Autodesk Inventor part; units mm, degrees
ref_plane "Work Plane1" through (16, 0, 0) normal (1, 0, 0) x (0, 1, 0)
ref_plane "XZ Plane" through (0, 0, 0) normal (0, 1, 0) x (-1, 0, 0)
ref_plane "XY Plane" through (0, 0, 0) normal (0, 0, 1) x (1, 0, 0)
sketch "Sketch1" plane through (0, 0, 0) normal (0, 0, 1) x (1, 0, 0)
  circle A0 centre (0, 0) radius 16
  circle A1 centre (0, 0) radius 14
  dimension "d0" = 32
  dimension "d3" = 28
extrude "Extrusion1" add sketch "Sketch1" along normal blind 300
ref_plane "Work Plane1" through (16, 0, 0) normal (1, 0, 0) x (0, 1, 0)
sketch "Sketch2" plane through (16, 0, 0) normal (1, 0, 0) x (0, 1, 0)
  circle A0 centre (0, 15) radius 4
  line L0 (0, -97.8) -> (0, 586.8)
  line L1 (16, 0) -> (-16, 0)
  circle A1 centre (0, 285) radius 4
  line L2 (16, 300) -> (-16, 300)
  point P0 (0, 0)
  dimension "d4" = 8
  dimension "d5" = 15
  dimension "d6" = 8
  dimension "d7" = 15
extrude "Extrusion2" cut sketch "Sketch2" against normal through all
properties part number "Steering PVC" material "PVC-Piping"
Here's how the part is built. I have some questions about the finished solid (model axes, mm). Coordinates: 2 decimals unless noted, no trailing zeros. Order: outer loops, then holes, each group sorted by start corner. A loop starts at its lowest first (then second) coordinate and runs counter-clockwise, first axis right, second up. Notation, with made-up numbers: (84, -38) -> (103, -38) arc R14 ccw to (103, -20) -> close; hole circle Ø1 at (-24, 60.25). An arc over 180 degrees is marked (long way). Answer in a Markdown table with one row per item.
(1) I want a section at B-B on y = 11.5. List the corners of the cut face in (x, z) for me, then the cut area to 3 significant figures.
Answer key:
| item | result |
|---|---|
| outline | (-11.12, 0) -> (-7.98, 0) -> (-7.98, 300) -> (-11.12, 300) -> close; (7.98, 0) -> (11.12, 0) -> (11.12, 300) -> (7.98, 300) -> close |
| area | 1,880 mm^2 |
(2) Please list where these lines run through material, in increasing order: probe 1 along Z at (x, y) = (15.1, 0); probe 2 along Y at (x, z) = (0, 102.5); probe 3 along Y at (x, z) = (2.5, 30.5).
Answer key:
| item | result |
|---|---|
| probe 1 | 0 to 11, 19 to 281, 289 to 300 |
| probe 2 | -16 to -14, 14 to 16 |
| probe 3 | -15.8 to -13.77, 13.77 to 15.8 |
(3) Thinking about a two-plate mould opening in Z: for faces 1 (the face through (-0.07, -14.15, 300)), 2 (the face through (14.726, -0.521, 18.966)), 3 (the face through (-0.07, -14.15, 0)), which applies, +Z half, -Z half, draft (parallel to the pull), parting line (faces both ways), or undercut?
Answer key:
| item | result |
|---|---|
| face 1 | +Z half |
| face 2 | undercut |
| face 3 | -Z half |
(4) I want a section at C-C on z = 116. List the corners of the cut face in (x, y) for me.
Answer key:
| item | result |
|---|---|
| outline | circle Ø32 at (0, 0); hole circle Ø28 at (0, 0) |
(5) Will these pins go through, and if not, where does the flat tip stop? pin 1 Ø3 at (x, z) = (2, 213.5) entering from +Y; pin 2 Ø5 at (x, y) = (-2, 12) entering from -Z; pin 3 Ø1.5 at (x, z) = (-7.5, 222) entering from +Y.
Answer key:
| item | result |
|---|---|
| pin 1 | y = 15.99 |
| pin 2 | z = 0 |
| pin 3 | y = 14.51 |
(6) I want a section at A-A on x = 0. List the corners of the cut face in (y, z) for me, then the cut area to 3 significant figures.
Answer key:
| item | result |
|---|---|
| outline | (-16, 0) -> (-14, 0) -> (-14, 300) -> (-16, 300) -> close; (14, 0) -> (16, 0) -> (16, 300) -> (14, 300) -> close |
| area | 1,200 mm^2 |
